Check sheet for the modelled part. Datum: model origin and axes. Units: mm. Face numbers are marked on the shaded views. A direction names the side the tool comes from. Round coordinates to 2 decimals unless told otherwise and drop trailing zeros. Order: outer loops, then holes, each group sorted by start corner. A loop starts at its lowest first (then second) coordinate and runs counter-clockwise, first axis right, second up.
(1) Sectioned sample at A-A, the plane x = -21. Enter the section's corners in (y, z) (3 decimals).
(2) Sectioned sample at D-D, the plane x = -15.5. Enter the section's corners in (y, z).
(3) Thickness scan on probe 1 along Y at (x, z) = (-17, 22); probe 2 along Z at (x, y) = (-0.5, -7); probe 3 along Z at (x, y) = (-21, 5). Record the ranges inside material, lowest first.
(4) Tool access check on the marked faces 1 and 2. Record the directions out of +Z, -Z, +X, -X, +Y, -Y that give a thin tool (end or side, any length) a straight path to the whole face; none if there is none.
(5) Depth check by flat-ended pin: pin 1 (6 mm diameter, centred on x = 11, z = 12, fed in from +Y); pin 2 (4.5 mm diameter, centred on y = 6.5, z = 2.5, fed in from +X). Enter the tip coordinate at first touch or a pass-through.
(6) Mould release check, pull along Y, two halves, no side actions. Record for the marked faces 3, 4 and 5: released by +Y, released by -Y, zero draft, split by the parting line, or undercut.
(7) Sectioned sample at B-B, the plane z = 3.5. Enter the section's corners in (x, y), and give its area (3 significant figures).
(8) Sectioned sample at C-C, the plane y = -38. Enter the section's corners in (x, z), and give its area (3 significant figures).
```python
from build123d import *

# Parameters (mm, degrees)
F0_W     = 50.8
F0_H     = 101.6
F1_DEPTH = 6.35
F2_W     = 50.8
F2_H     = 2.54
F3_DEPTH = 38.1
F6_DEPTH = 6.35
F7_DEPTH = 6.35


with BuildPart() as f1:
    # F0 (on Top) → F1 (new body)
    with BuildSketch(Plane.XY):
        Rectangle(F0_W, F0_H)
    extrude(amount=F1_DEPTH)

    # F2 (on face) → F3 (join)
    with BuildSketch(Plane.XY.offset(6.35)):
        with Locations((0, -49.53)):
            Rectangle(F2_W, F2_H)
    extrude(amount=F3_DEPTH)

    # F5 (on face) → F6 (cut)
    with BuildSketch(Plane.YZ.offset(25.4)):
        with BuildLine():
            Line((-0.7833918417, 0), (21.1033918417, 0))
            ThreePointArc((21.1033918417, 0), (10.16, 5.715), (-0.7833918417, 0))
        make_face()
    extrude(amount=-F6_DEPTH, mode=Mode.SUBTRACT)

    # F4 (on face) → F7 (cut)
    with BuildSketch(Plane(origin=(-25.4, 0, 0), x_dir=(0, -1, 0), z_dir=(-1, 0, 0))):
        with BuildLine():
            Line((-21.1033918417, 0), (0.7833918417, 0))
            ThreePointArc((0.7833918417, 0), (-10.16, 5.715), (-21.1033918417, 0))
        make_face()
    extrude(amount=-F7_DEPTH, mode=Mode.SUBTRACT)


solid = f1.part
```
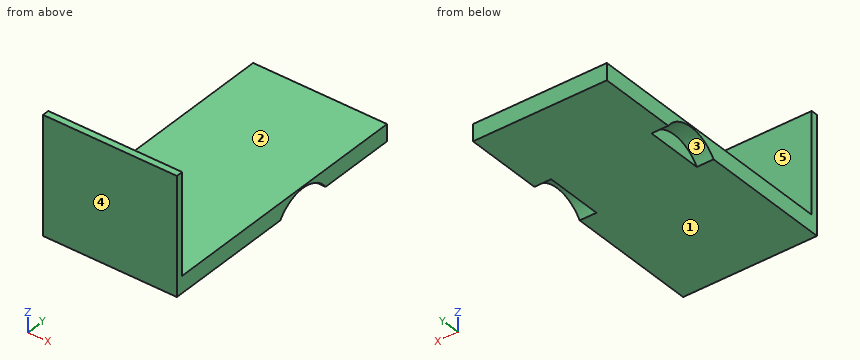
Derived:
1. outline: (-50.8, 0) - (-0.783, 0) arc R13.335 cw to (21.103, 0) - (50.8, 0) - (50.8, 6.35) - (-48.26, 6.35) - (-48.26, 44.45) - (-50.8, 44.45) - close
2. outline: (-50.8, 0) - (50.8, 0) - (50.8, 6.35) - (-48.26, 6.35) - (-48.26, 44.45) - (-50.8, 44.45) - close
3. probe 1: y = -50.8 to -48.26
3. probe 2: z = 0 to 6.35
3. probe 3: z = 4.68 to 6.35
4. face 1: -Z, +X, -X, +Y, -Y
4. face 2: +Z, +X, -X, +Y
5. pin 1: stops at y = -48.26
5. pin 2: stops at x = 19.05
6. face 3: undercut
6. face 4: released by -Y
6. face 5: released by +Y
7. outline: (-25.4, -50.8) - (25.4, -50.8) - (25.4, 2.8) - (19.05, 2.8) - (19.05, 17.52) - (25.4, 17.52) - (25.4, 50.8) - (-25.4, 50.8) - (-25.4, 17.52) - (-19.05, 17.52) - (-19.05, 2.8) - (-25.4, 2.8) - close
7. area: 4,970 mm2
8. outline: (-25.4, 0) - (25.4, 0) - (25.4, 6.35) - (-25.4, 6.35) - close
8. area: 323 mm2
